from build123d import *

# Parameters (mm, degrees)
SKETCH1_R           = 2
SKETCH1_R_2         = 38.03346271
BOSS_EXTRUDE1_DEPTH = 4
FILLET1_R           = 2


with BuildPart() as part:
    # Sketch1 → Boss-Extrude1 (new body)
    with BuildSketch(Plane.XY):
        Polygon((0, 0), (9, 0), (9, 5), (75, 5), (74.999999866, -2.502e-06), (84, 0), (84, -7.5), (87, -7.5), (87, -2.5), (90, -2.5), (90, -82.5), (87, -82.5), (87, -77.5), (84, -77.5), (84, -85.000002502), (74.999993421, -85.000002502), (74.999993042, -90.000002502), (9, -90), (9, -85), (0, -85), (0, -77.5), (-3, -77.5), (-3, -82.5), (-6, -82.5), (-6, -2.5), (-3, -2.5), (-3, -7.5), (0, -7.5), align=None)
        with Locations((4, -5.500026536)):
            Circle(SKETCH1_R, mode=Mode.SUBTRACT)
        with Locations((80.000043308, -5.499945424)):
            Circle(SKETCH1_R, mode=Mode.SUBTRACT)
        with Locations((80, -79.499973464)):
            Circle(SKETCH1_R, mode=Mode.SUBTRACT)
        with Locations((3.999956692, -79.500054576)):
            Circle(SKETCH1_R, mode=Mode.SUBTRACT)
        with Locations((41.999998297, -43.155631615)):
            Circle(SKETCH1_R_2, mode=Mode.SUBTRACT)
    extrude(amount=BOSS_EXTRUDE1_DEPTH)

    # Fillet1
    fillet1_edges = [part.edges().sort_by_distance(p)[0] for p in [
        (3.966535587, -43.155631615, 0),
        (3.966535587, -43.155631615, 4),
    ]]
    fillet(fillet1_edges, radius=FILLET1_R - 0.0001)  # a hair under: the kernel refuses the full size


solid = part.part
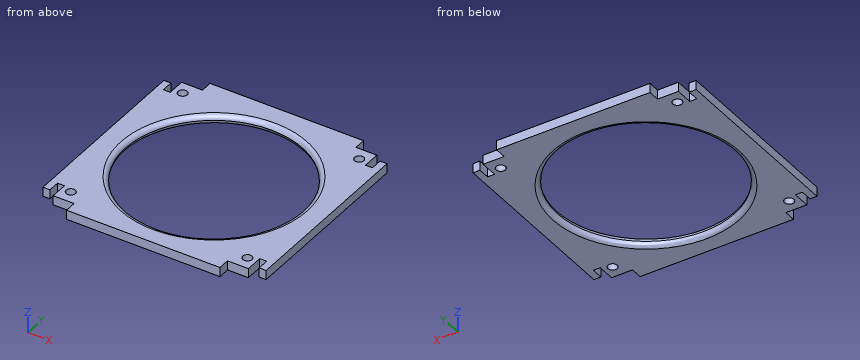
The model under review builds one solid part; all positions refer to its coordinate system, in mm. Round coordinates to 2 decimals unless told otherwise and drop trailing zeros. Return JSON: item names as keys, results as strings.
(1) For pin 1 (2 mm diameter, centred on x = 81.5, z = 3, fed in from +Y); pin 2 (2 mm diameter, centred on y = 1.5, z = 2, fed in from -X); pin 3 (1.2 mm diameter, centred on x = 78, z = 2.5, fed in from -Y), all flat-tipped, find the tip position at first contact; note any pin that passes through.
Solved:
{"pin 1": "y = 0", "pin 2": "x = 9", "pin 3": "y = -85"}
(2) Add section A-A on z = 1.35. State how many separate pieces and enclosed holes the cut face has, plus the area to 3 significant figures.
Solved:
{"separate pieces": "1", "enclosed holes": "5", "area": "4,080 mm2"}
(3) For line 1 (X direction, y = -38.5, z = 3); line 2 (Y direction, x = 81.5, z = 2.2); line 3 (Y direction, x = 17.5, z = 1.75), list the stretches that pass through material, from the lowest coordinate up.
Solved:
{"line 1": "-6 to 3.98, 80.02 to 90", "line 2": "-85 to -80.82, -78.18 to -6.82, -4.18 to 0", "line 3": "-90 to -72.27, -14.04 to 5"}
